Autodesk Fusion 360 part; units mm, degrees
sketch "Sketch1" plane through (0, 0, 0) normal (0, 0, 1) x (1, 0, 0)
  line L0 (-100, 50) -> (100, 50)
  line L1 (100, 50) -> (100, -50)
  line L2 (100, -50) -> (-100, -50)
  line L3 (-100, -50) -> (-100, 50)
  line L4 (-100, 50) -> (100, -50) construction
  line L5 (100, 50) -> (-100, -50) construction
  line L6 (-55, 37.5) -> (55, 37.5)
  line L7 (75, 17.5) -> (75, -17.5)
  line L8 (55, -37.5) -> (-55, -37.5)
  line L9 (-75, -17.5) -> (-75, 17.5)
  line L10 (-75, 37.5) -> (75, -37.5) construction
  line L11 (75, 37.5) -> (-75, -37.5) construction
  arc A0 (-55, 37.5) -> (-75, 17.5) centre (-55, 17.5) ccw
  arc A1 (-75, -17.5) -> (-55, -37.5) centre (-55, -17.5) ccw
  arc A2 (55, -37.5) -> (75, -17.5) centre (55, -17.5) ccw
  arc A3 (75, 17.5) -> (55, 37.5) centre (55, 17.5) ccw
  circle A4 centre (0, 0) radius 25
  dimension "d1" = 200
  dimension "d2" = 100
  dimension "d3" = 150
  dimension "d4" = 75
  dimension "d5" = 20
  dimension "d6" = 20
  dimension "d7" = 50
extrude "Extrude1" add sketch "Sketch1" along normal blind 20 contours L0 L1 L2 L3
extrude "Extrude2" add sketch "Sketch1" along normal blind 10 contours L6 L7 L8 L9 A0 A1 A2 A3
extrude "Extrude3" add sketch "Sketch1" along normal blind 20 contours A4
Can you work these out from the model? Positions are in its coordinate system, mm. A direction names the side the tool comes from. Coordinates: 2 decimals unless noted, no trailing zeros. Loops run counter-clockwise (first coordinate to the right, second up) from the corner with the lowest first, then second, coordinate; pieces in that order, holes last.
1) Imagine slicing it at C-C on y = 0. List the corners of the cut face in (x, z) for me, plus the area to 3 significant figures.
2) Which directions (+Z, -Z, +X, -X, +Y, -Y) give clear straight access to the entire face, cutting with the end or side of a thin tool? Please do faces 5 (the flat face through (1, -37.5, 15)), 6 (the flat face through (-1, 50, 10)).
3) Imagine slicing it at D-D on x = -70. List the corners of the cut face in (y, z) for me.
4) Imagine slicing it at A-A on z = 15.75. List the corners of the cut face in (x, y) for me.
5) For pin 1 (1.5 mm diameter, centred on x = -28.5, y = -17.5, fed in from +Z), with a flat end and sliding along its axis, tell me the tip position at first contact or that it passes through.
6) Thinking about a two-plate mould opening in X: for faces 1 (the cylindrical face through (23.846, -7.509, 14.93)), 2 (the flat face through (1, -50, 10)), 3 (the flat face through (100, 1, 10)), 4 (the flat face through (-1, 37.5, 15)), which applies, pulls with the +X half, pulls with the -X half, needs draft (parallel to the pull), parting line crosses it, or undercut?
7) Imagine slicing it at B-B on x = -45. List the corners of the cut face in (y, z) for me.
8) I need wall thicknesses on probe 1 along X at (y, z) = (1, 10.25); probe 2 along Y at (x, z) = (-53.5, 17.25); probe 3 along X at (y, z) = (21.5, 14.5). Which ranges of each line are inside material? Lowest first, please.
Completed:
1. outline: (-100, 0) - (100, 0) - (100, 20) - (75, 20) - (75, 10) - (25, 10) - (25, 20) - (-25, 20) - (-25, 10) - (-75, 10) - (-75, 20) - (-100, 20) - close
1. area: 3,000 mm2
2. face 5: +Z
2. face 6: +Z, -Z, +X, -X, +Y
3. outline: (-50, 0) - (50, 0) - (50, 20) - (30.73, 20) - (30.73, 10) - (-30.73, 10) - (-30.73, 20) - (-50, 20) - close
4. outline: (-100, -50) - (100, -50) - (100, 50) - (-100, 50) - close; circle Ø50 at (0, 0); hole (-75, -17.5) arc R20 ccw to (-55, -37.5) - (55, -37.5) arc R20 ccw to (75, -17.5) - (75, 17.5) arc R20 ccw to (55, 37.5) - (-55, 37.5) arc R20 ccw to (-75, 17.5) - close
5. pin 1: stops at z = 10
6. face 1: undercut
6. face 2: needs draft
6. face 3: pulls with the +X half
6. face 4: undercut
7. outline: (-50, 0) - (50, 0) - (50, 20) - (37.5, 20) - (37.5, 10) - (-37.5, 10) - (-37.5, 20) - (-50, 20) - close
8. probe 1: x = -100 to -75, -24.98 to 24.98, 75 to 100
8. probe 2: y = -50 to -37.5, 37.5 to 50
8. probe 3: x = -100 to -74.6, -12.76 to 12.76, 74.6 to 100
